```python
from build123d import *

# Parameters (mm, degrees)
F0_W      = 40
F0_H      = 30
F1_DEPTH  = 2
F2_R      = 1.75
F3_DEPTH  = 5
F4_R      = 1.75
F5_DEPTH  = 5
F7_DEPTH  = 2.001
F8_W      = 100
F8_H      = 50
F9_DEPTH  = 2
F10_R     = 5
F11_DEPTH = 2.001
F12_W     = 8
F12_H     = 20
F13_DEPTH = 10
F14_W     = 8
F14_H     = 8.75
F15_DEPTH = 2
F16_R     = 1.75
F17_DEPTH = 5
F18_R     = 1.75
F19_DEPTH = 7.001
F20_R     = 10


with BuildPart() as f1:
    # F0 (on Top) → F1 (new body)
    with BuildSketch(Plane.XY):
        with Locations((0, 12.5)):
            Rectangle(F0_W, F0_H)
    extrude(amount=F1_DEPTH)

    # F2 (on face) → F3 (join)
    with BuildSketch(Plane.XY.offset(2)):
        with Locations((14.7, 0)):
            Circle(F2_R)
        with Locations((-14.7, 0)):
            Circle(F2_R)
    extrude(amount=F3_DEPTH)

    # F4 (on face) → F5 (join)
    with BuildSketch(Plane.XY.offset(2)):
        with Locations((-4.7, 20)):
            Circle(F4_R)
        with Locations((4.7, 20)):
            Circle(F4_R)
    extrude(amount=F5_DEPTH)

    # F6 (on face) → F7 (cut, through all)
    with BuildSketch(Plane.XY.offset(2)):
        with BuildLine():
            ThreePointArc((-14.3824583655, 17.5), (-14.2570409722, 22.9432920101), (-11.298423737, 27.5140404701))
            Line((-11.298423737, 27.5140404701), (-20, 27.5140404701))
            Line((-20, 27.5140404701), (-20, 17.5))
            Line((-20, 17.5), (-14.3824583655, 17.5))
        make_face()
        with BuildLine():
            Line((20, 27.5140404701), (11.298423737, 27.5140404701))
            ThreePointArc((11.298423737, 27.5140404701), (14.2570409722, 22.9432920101), (14.3824583655, 17.5))
            Line((14.3824583655, 17.5), (20, 17.5))
            Line((20, 17.5), (20, 27.5140404701))
        make_face()
    extrude(amount=-F7_DEPTH, mode=Mode.SUBTRACT)

    # F8 (on Top) → F9 (join)
    with BuildSketch(Plane.XY):
        with Locations((0, -27.5)):
            Rectangle(F8_W, F8_H)
    extrude(amount=F9_DEPTH)

    # F10 (on face) → F11 (cut, through all)
    with BuildSketch(Plane.XY.offset(2)):
        with Locations((-14.7, -29)):
            Circle(F10_R)
    extrude(amount=-F11_DEPTH, mode=Mode.SUBTRACT)

    # F12 (on face) → F13 (join)
    with BuildSketch(Plane(origin=(0, 0, 0), x_dir=(1, 0, 0), z_dir=(0, 0, -1))):
        with Locations((-29, 28.5)):
            Rectangle(F12_W, F12_H)
        with Locations((19, 28.5)):
            Rectangle(F12_W, F12_H)
    extrude(amount=F13_DEPTH)

    # F14 (on face) → F15 (join)
    with BuildSketch(Plane(origin=(0, 0, -10), x_dir=(1, 0, 0), z_dir=(0, 0, -1))):
        with Locations((-29, 22.875)):
            Rectangle(F14_W, F14_H)
        with Locations((-29, 34.125)):
            Rectangle(F14_W, F14_H)
        with Locations((19, 34.125)):
            Rectangle(F14_W, F14_H)
        with Locations((19, 22.875)):
            Rectangle(F14_W, F14_H)
    extrude(amount=F15_DEPTH)

    # F16 (on face) → F17 (cut)
    with BuildSketch(Plane(origin=(0, 0, -12), x_dir=(1, 0, 0), z_dir=(0, 0, -1))):
        with Locations((-29.1, 33.5)):
            Circle(F16_R)
        with Locations((-29.1, 23.5)):
            Circle(F16_R)
        with Locations((19.1, 23.5)):
            Circle(F16_R)
        with Locations((19.1, 33.5)):
            Circle(F16_R)
    extrude(amount=-F17_DEPTH, mode=Mode.SUBTRACT)

    # F18 (on face) → F19 (cut, through all)
    with BuildSketch(Plane(origin=(0, 0, 0), x_dir=(1, 0, 0), z_dir=(0, 0, -1))):
        Polygon((-38, 52.5), (-50, 52.5), (-50, 47.5), (-50, 2.5), (-38, 2.5), (-38, 47.5), (38, 47.5), (38, 2.5), (50, 2.5), (50, 47.5), (50, 52.5), (38, 52.5), align=None)
        with Locations((-5, 44)):
            Circle(F18_R)
        with Locations((5, 44)):
            Circle(F18_R)
    extrude(amount=-F19_DEPTH, mode=Mode.SUBTRACT)

    # F20
    f20_edges = [f1.edges().sort_by_distance(p)[0] for p in [
        (-38, -2.5, 1),
        (38, -2.5, 1),
        (-38, -47.5, 1),
        (38, -47.5, 1),
    ]]
    fillet(f20_edges, radius=F20_R)


solid = f1.part
```
Verification items for the finished model (mm, model axes). A direction names the side the tool comes from. Give positions to 0.01 mm unless a question says otherwise; leave off trailing zeros. Loops run counter-clockwise (first coordinate to the right, second up) from the corner with the lowest first, then second, coordinate; pieces in that order, holes last. Notation, with made-up numbers: M 35.25,74.25 L 54.25,74.25 A20 cw 54.25,109.25 Z; hole C 1.25,74 d4. An arc over 180 degrees is marked long. Return JSON: item names as keys, results as strings.
1) Material ranges on L1, parallel to Y at x = -29.1, z = -8.85; L2, parallel to X at y = -33.5, z = -8.8; L3, parallel to Y at x = 5, z = 0.8, recorded low to high. Write a range as [from, to].
Findings:
{"L1": "y = [-38.5, -35.25], [-31.75, -25.25], [-21.75, -18.5]", "L2": "x = [-33, -30.85], [-27.35, -25], [15, 17.35], [20.85, 23]", "L3": "y = [-47.5, -45.75], [-42.25, 27.5]"}
2) Section check D-D, the plane x = -29.1. Enter the section's corners in (y, z), and give its area (3 significant figures).
Findings:
{"outline": "M -47.44,0 L -38.5,0 L -38.5,-12 L -35.25,-12 L -35.25,-7 L -31.75,-7 L -31.75,-12 L -29.75,-12 L -29.75,-10 L -27.25,-10 L -27.25,-12 L -25.25,-12 L -25.25,-7 L -21.75,-7 L -21.75,-12 L -18.5,-12 L -18.5,0 L -2.56,0 L -2.56,2 L -47.44,2 Z", "area": "290 mm2"}
3) Section check C-C, the plane x = -4.7. Enter the section's corners in (y, z), and give its area (3 significant figures).
Findings:
{"outline": "M -47.5,0 L -45.72,0 L -45.72,2 L -47.5,2 Z; M -42.28,0 L 27.5,0 L 27.5,2 L 21.75,2 L 21.75,7 L 18.25,7 L 18.25,2 L -42.28,2 Z", "area": "161 mm2"}
4) Gauge pin test, flat ends, axial feed: P1, Ø6, axis at x = -14, y = 10.5, coming from the +Z side; P2, Ø6, axis at y = -31, z = -4.5, coming from the -X side; P3, Ø3, axis at x = -7, z = 2.5, coming from the +Y side; P4, Ø1, axis at y = 7.5, z = 1, coming from the -X side. Record the tip position at first contact, or that the pin passes through.
Findings:
{"P1": "stops at z = 2", "P2": "stops at x = -33", "P3": "stops at y = 27.5", "P4": "stops at x = -20"}
5) Section check B-B, the plane y = 0. Enter the section's corners in (x, z).
Findings:
{"outline": "M -20,0 L 20,0 L 20,2 L 16.45,2 L 16.45,7 L 12.95,7 L 12.95,2 L -12.95,2 L -12.95,7 L -16.45,7 L -16.45,2 L -20,2 Z"}
6) Tool access check on faces 1 (the cylindrical face through (-4.928, 21.735, 4.465)), 2 (the flat face through (-29, -34, -7)), 3 (the flat face through (19, -29.75, -11)), 4 (the flat face through (-25, -28, -6)), 5 (the flat face through (-33, -28, -6)). Record the directions out of +Z, -Z, +X, -X, +Y, -Y that give a thin tool (end or side, any length) a straight path to the whole face; none if there is none.
Findings:
{"face 1": "+Z", "face 2": "-Z", "face 3": "-Z, +X, -X", "face 4": "-Z, +Y, -Y", "face 5": "-Z, -X, +Y, -Y"}
7) Section check A-A, the plane z = -4.75. Enter the section's corners in (x, y), and give its area (3 significant figures).
Findings:
{"outline": "M -33,-38.5 L -25,-38.5 L -25,-18.5 L -33,-18.5 Z; M 15,-38.5 L 23,-38.5 L 23,-18.5 L 15,-18.5 Z", "area": "320 mm2"}
8) Mould release check, pull along Y, two halves, no side actions. Record for faces 6 (the cylindrical face through (20.769, -34.026, -9.535)), 7 (the flat face through (-29, -18.5, -6)), 8 (the flat face through (0, -47.5, 1)), 9 (the flat face through (-29, -27.25, -11)): released by +Y, released by -Y, zero draft, split by the parting line, or undercut.
Findings:
{"face 6": "undercut", "face 7": "released by +Y", "face 8": "released by -Y", "face 9": "undercut"}
